```python
from build123d import *

# Parameters (mm, degrees)
SKETCH1_R           = 3.175
SKETCH1_W           = 4.953
SKETCH1_H           = 6.35
BOSS_EXTRUDE1_DEPTH = 2.4765


with BuildPart() as part:
    # Sketch1 → Boss-Extrude1 (new, symmetric)
    with BuildSketch(Plane(origin=(0, 0, 0), x_dir=(0, 0, -1), z_dir=(1, 0, 0))):
        with BuildLine():
            Line((-94.642365809, 54.483), (-122.457292876, 54.483))
            Line((-122.457292876, 54.483), (-122.457292876, 49.53))
            Line((-122.457292876, 49.53), (-142.309833129, 39.889958968))
            ThreePointArc((-142.309833129, 39.889958968), (-159.075906045, 45.361766519), (-154.207292876, 62.312827982))
            Line((-154.207292876, 62.312827982), (-115.855925951, 84.455))
            Line((-115.855925951, 84.455), (20.203427503, 84.455))
            Line((20.203427503, 84.455), (45.72, 69.723))
            Line((45.72, 69.723), (45.72, 49.403))
            Line((45.72, 49.403), (38.1, 49.403))
            Line((38.1, 49.403), (38.1, 54.483))
            Line((38.1, 54.483), (-10.2235, 54.483))
            Line((-10.2235, 54.483), (-10.2235, 60.833))
            Line((-10.2235, 60.833), (-15.1765, 60.833))
            Line((-15.1765, 60.833), (-15.1765, 54.483))
            Line((-15.1765, 54.483), (-21.651856626, 54.483))
            Line((-21.651856626, 54.483), (-21.651856626, 49.403))
            Line((-21.651856626, 49.403), (-29.271856626, 49.403))
            Line((-29.271856626, 49.403), (-29.271856626, 67.183))
            Line((-29.271856626, 67.183), (-87.022365809, 67.183))
            Line((-87.022365809, 67.183), (-87.022365809, 49.403))
            Line((-87.022365809, 49.403), (-94.642365809, 49.403))
            Line((-94.642365809, 49.403), (-94.642365809, 54.483))
        make_face()
        with Locations((-147.857292876, 51.314305354)):
            Circle(SKETCH1_R, mode=Mode.SUBTRACT)
        with Locations((-12.7, 73.66)):
            Rectangle(SKETCH1_W, SKETCH1_H, mode=Mode.SUBTRACT)
    extrude(amount=BOSS_EXTRUDE1_DEPTH, both=True)


solid = part.part
```
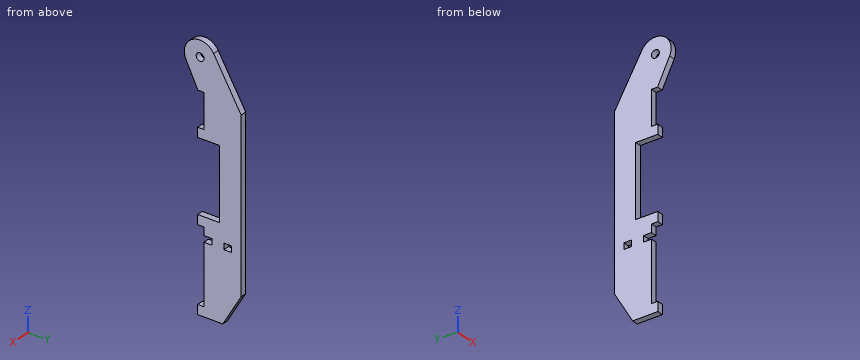
Could you check a few things on this model? Use its own coordinates, in mm. Coordinates: 2 decimals unless noted, no trailing zeros. Order: outer loops, then holes, each group sorted by start corner. A loop starts at its lowest first (then second) coordinate and runs counter-clockwise, first axis right, second up. Notation, with made-up numbers: M -11.75,8 L 46.25,8 A23 cw 46.25,24 Z; hole C -10,14 d4. An arc over 180 degrees is marked long. Use a Markdown table: item, result. Add a question column.
Q1. I want a section at D-D on y = 74.5. List the corners of the cut face in (x, z) for me.
Q2. I want a section at A-A on x = 0.95. Give the number of separate pieces and of enclosed holes in the cut face, then the cut area to 3 significant figures.
Q3. I want a section at C-C on z = -10. List the corners of the cut face in (x, y) for me (1 decimal).
Q4. If I drill on L1, parallel to Z at x = -1.65, y = 51.5; L2, parallel to Y at x = 1.75, z = 13.5 (3 decimals); L3, parallel to Y at x = 0.1, z = 35 (3 decimals), over which ranges is the centre line in solid material (lowest first)?
Q5. I want a section at B-B on y = 64.5. List the corners of the cut face in (x, z) for me, then the cut area to 3 significant figures.
Q6. I'm going to push flat-ended pins straight in: pin 1 (2.5 mm diameter, centred on x = 0.5, z = 91, fed in from -Y); pin 2 (5.5 mm diameter, centred on y = 51.31, z = 147.86, fed in from +X); pin 3 (2.5 mm diameter, centred on x = 0, z = 13.5, fed in from -Y); pin 4 (2 mm diameter, centred on x = 1.5, y = 71.5, fed in from +Z). Where does each tip first touch, or does it pass through?
Checked values:
| question | item | result |
|---|---|---|
| 1 | outline | M -2.48,-37.45 L 2.48,-37.45 L 2.48,10.22 L -2.48,10.22 Z; M -2.48,15.18 L 2.48,15.18 L 2.48,133.1 L -2.48,133.1 Z |
| 2 | separate pieces | 1 |
| 2 | enclosed holes | 2 |
| 2 | area | 5,140 mm² |
| 3 | outline | M -2.5,54.5 L 2.5,54.5 L 2.5,84.5 L -2.5,84.5 Z |
| 4 | L1 | -45.72 to -38.1, 21.65 to 29.27, 87.02 to 94.64, 122.46 to 144.69, 151.03 to 160.56 |
| 4 | L2 | 60.833 to 70.485, 76.835 to 84.455 |
| 4 | L3 | 67.183 to 84.455 |
| 5 | outline | M -2.48,-45.72 L 2.48,-45.72 L 2.48,29.27 L -2.48,29.27 Z; M -2.48,87.02 L 2.48,87.02 L 2.48,150.42 L -2.48,150.42 Z |
| 5 | area | 685 mm² |
| 6 | pin 1 | y = 49.4 |
| 6 | pin 2 | through |
| 6 | pin 3 | y = 60.83 |
| 6 | pin 4 | z = 140.03 |
